Job drawing, mm, ordinate dimensions from the low corner. One solid piece. A direction names the side the tool comes from. Round coordinates to 2 decimals unless told otherwise and drop trailing zeros. Loops run counter-clockwise (first coordinate to the right, second up) from the corner with the lowest first, then second, coordinate; pieces in that order, holes last. Notation, with made-up numbers: M 44,14.5 L 78,14.5 A22 ccw 78,46.5 Z; hole C 41,81.25 d2. An arc over 180 degrees is marked long. Put each result on its own line as item: value. Start each with the question number.
1) Drop flat-ended pins along their axis: pin 1 Ø4 at (x, y) = (20.75, 20.87) entering from +Z; pin 2 Ø10 at (x, y) = (21, 5.5) entering from -Z; pin 3 Ø2 at (x, z) = (21.5, 20.5) entering from +Y. Give the stop position or say it passes through.
2) Slice it at C-C on z = 20.75. Give the cut face in (x, y).
3) Probe line 1 along Y through (x, z) = (20.75, 25.05); line 2 along Y through (x, z) = (20.75, 38) (1 decimal); line 3 along Z through (x, y) = (19.5, 28). List the from-to ranges inside material, lowest first.
4) Pull direction Z, two halves, no side cores. Call the marked faces 3, 4, 5 and 6: +Z half, -Z half, draft (parallel to the pull), parting line (faces both ways), or undercut.
5) Slice it at A-A on x = 21. Give the cut face in (y, z).
6) Which spindle directions (+Z, -Z, +X, -X, +Y, -Y) get a long thin tool onto all of the face, cutting with end or side? Do the marked faces 1 and 2. Say none if no direction does.
7) Slice it at D-D on x = 27. Give the cut face in (y, z).
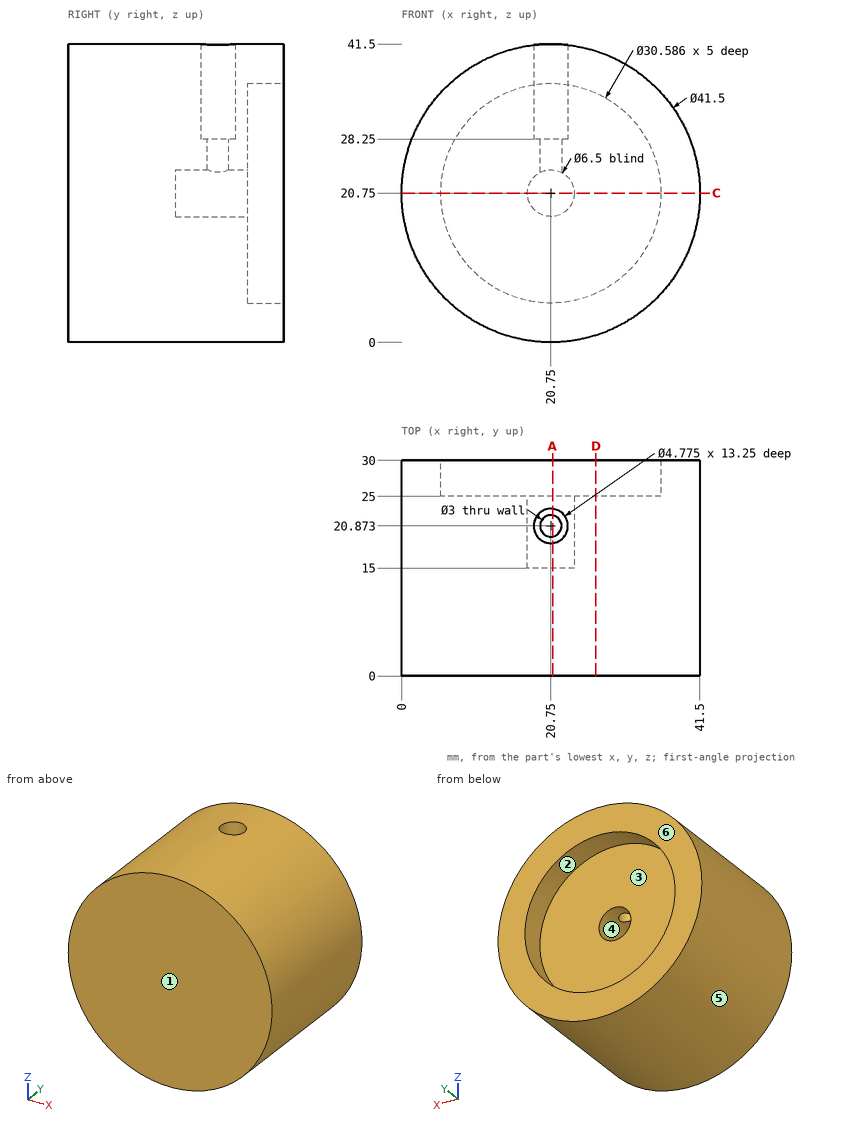
Recorded:
1. pin 1: stops at z = 28.25
1. pin 2: stops at z = 0
1. pin 3: stops at y = 15
2. outline: M 0,0 L 41.5,0 L 41.5,30 L 36.04,30 L 36.04,25 L 24,25 L 24,15 L 17.5,15 L 17.5,25 L 5.46,25 L 5.46,30 L 0,30 Z
3. line 1: y = 0 to 19.37, 22.37 to 25
3. line 2: y = 0 to 18.5, 23.3 to 30
3. line 3: z = 0.04 to 5.51, 35.99 to 41.46
4. face 3: undercut
4. face 4: undercut
4. face 5: parting line
4. face 6: draft
5. outline: M 0,0 L 30,0 L 30,5.46 L 25,5.46 L 25,17.51 L 15,17.51 L 15,23.99 L 19.39,23.99 L 19.39,28.25 L 18.5,28.25 L 18.5,41.5 L 0,41.5 Z; M 22.35,23.99 L 25,23.99 L 25,36.04 L 30,36.04 L 30,41.5 L 23.25,41.5 L 23.25,28.25 L 22.35,28.25 Z
6. face 1: +Z, -Z, +X, -X, -Y
6. face 2: +Y
7. outline: M 0,0.96 L 30,0.96 L 30,6.79 L 25,6.79 L 25,34.71 L 30,34.71 L 30,40.54 L 0,40.54 Z
